Check sheet for the modelled part. Datum: model origin and axes. Units: mm. Face numbers are marked on the shaded views. A direction names the side the tool comes from. Give positions to 0.01 mm unless a question says otherwise; leave off trailing zeros. Write each loop counter-clockwise with the first axis right and the second up, starting at its lowest first coordinate (ties: lowest second). Pieces come first, ordered by that corner, then holes. Notation, with made-up numbers: M 61.5,-19 L 99.5,-19 A10 cw 99.5,0 Z; hole C -34,-13 d8. An arc over 180 degrees is marked long. Use CSV: the item, a comma, the result in double quotes. Start each with the question number.
1. Cross-section at C-C, the plane y = 12. Enter the section's corners in (x, z).
2. Cross-section at B-B, the plane x = 9. Enter the section's corners in (y, z).
3. Depth check by flat-ended pin: P1, Ø7.5, axis at x = -22.5, y = 13.5, coming from the +Z side; P2, Ø0.9, axis at x = -9, z = -18, coming from the +Y side; P3, Ø2.5, axis at x = -9.85, z = -18.519, coming from the -Y side; P4, Ø2, axis at y = -6.547, z = -15, coming from the -X side. Enter the tip coordinate at first touch or a pass-through.
4. Mould release check, pull along Z, two halves, no side actions. Record for the marked faces 6, 7, 8 and 9: +Z half, -Z half, draft (parallel to the pull), parting line (faces both ways), or undercut.
5. Access from +Z, -Z, +X, -X, +Y, -Y to the whole of each face (thin tool, end or side, straight path). Record for the marked faces 1, 2, 3, 4 and 5.
6. Cross-section at D-D, the plane y = -3.5. Enter the section's corners in (x, z).
7. Scan lines: line 1 (X direction, y = 2.45, z = -15); line 2 (X direction, y = 35.5, z = -11); line 3 (Y direction, x = -23, z = -21). Record each from-to range of solid material in increasing order.
8. Cross-section at A-A, the plane x = -17. Enter the section's corners in (y, z).
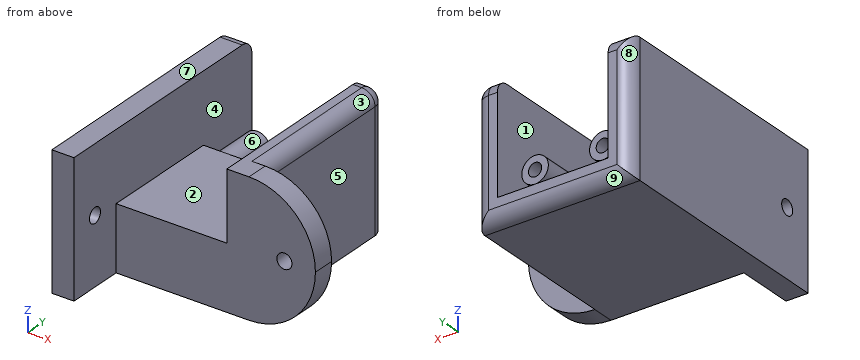
Autodesk Inventor part; units mm, degrees
ref_plane "YZ Plane" through (0, 0, 0) normal (1, 0, 0) x (0, 1, 0)
ref_plane "XZ Plane" through (0, 0, 0) normal (0, 1, 0) x (-1, 0, 0)
ref_plane "XY Plane" through (0, 0, 0) normal (0, 0, 1) x (1, 0, 0)
sketch "Sketch1" plane through (0, 0, 0) normal (0, 1, 0) x (-1, 0, 0)
  line L0 (0, 0) -> (35, 0) construction
  line L1 (35, 0) -> (35, -30)
  line L2 (35, -30) -> (0, -30)
  line L3 (0, -30) -> (0, 0)
  line L4 (30, -25) -> (30, -5)
  line L5 (30, -5) -> (5, -5) construction
  line L6 (5, -5) -> (5, -25)
  line L7 (5, -25) -> (30, -25)
  line L8 (30, -5) -> (30, 0)
  line L9 (5, -5) -> (5, 0)
  line L10 (5, 0) -> (0, 0)
  line L11 (30, 0) -> (35, 0)
  dimension "d0" = 35
  dimension "d1" = 30
  dimension "d2" = 5
extrude "Extrusion1" add sketch "Sketch1" along normal blind 42
sketch "Sketch2" plane through (0, 0, 0) normal (0, 1, 0) x (-1, 0, 0)
  line L0 (30, 0) -> (30, -25)
  line L1 (5, -25) -> (5, 0)
  line L2 (30, -25) -> (5, -25)
  line L3 (5, -25) -> (5, -15.519)
  line L4 (5, -15.519) -> (30, -15.519)
  line L5 (30, -15.519) -> (30, -25)
  point P0 (0, 0)
  dimension "d5" = 9.481
extrude "Extrusion2" add sketch "Sketch2" along normal blind 27
sketch "Sketch3" plane through (0, 27, 0) normal (0, 1, 0) x (1, 0, 0)
  circle A0 centre (-25.15, 18.519) radius 1.5
  line L0 (-30, 0) -> (-30, 15.519)
  circle A1 centre (-25.15, 18.519) radius 3
  line L1 (-30, 15.519) -> (-5, 15.519)
  line L2 (-17.5, 15.519) -> (-17.5, 30) construction
  line L3 (0, 30) -> (-35, 30) construction
  circle A2 centre (-9.85, 18.519) radius 1.5
  circle A3 centre (-9.85, 18.519) radius 3
  point P0 (0, 0)
  dimension "d8" = 3
  dimension "d9" = 4.85
  dimension "d10" = 6
extrude "Extrusion3" add sketch "Sketch3" along normal blind 10
sketch "Sketch4" plane through (0, 0, 0) normal (0, -1, 0) x (1, 0, 0)
  line L0 (-35, -30) -> (-35, 0)
  line L1 (0, -30) -> (-35, -30)
  line L2 (-35, 0) -> (-30, 0)
  line L3 (-30, 0) -> (-30, -30)
  line L4 (-30, -30) -> (-35, -30)
  line L5 (-35, -30) -> (-35, 0)
  line L6 (-30, 0) -> (-30, -15.519)
  point P0 (0, 0)
extrude "Extrusion4" add sketch "Sketch4" along normal blind 13.047
sketch "Sketch5" plane through (0, 0, 0) normal (1, 0, 0) x (0, 0, -1)
  line L0 (15.519, 0) -> (0, 0)
  line L1 (30, 0) -> (30, 42)
  line L2 (0, 0) -> (30, 0)
  line L3 (30, 0) -> (30, 5)
  line L4 (30, 5) -> (0, 5)
  line L5 (0, 5) -> (0, 0)
  dimension "d15" = 5
extrude "Extrusion5" add sketch "Sketch5" along normal blind 15
sketch "Sketch6" plane through (0, 5, 0) normal (0, 1, 0) x (1, 0, 0)
  circle A0 centre (8, 7) radius 3.5 construction
  circle A1 centre (8, 23) radius 3.5 construction
  line L0 (8, 7) -> (8, 23) construction
  line L1 (8, 15) -> (15, 15) construction
  line L2 (15, 0) -> (15, 30) construction
  line L3 (15, 30) -> (15, 0) construction
  line L4 (0, 30) -> (15, 30) construction
  circle A2 centre (8, 15) radius 1.7
  point P0 (0, 0)
  dimension "d18" = 7
  dimension "d19" = 7
  dimension "d20" = 7
  dimension "d21" = 7
  dimension "d25" = 3.4
extrude "Extrusion6" cut sketch "Sketch6" against normal up to surface (5 mm away) from surface at 0
sketch "Sketch7" plane through (-35, 42, -30) normal (-1, 0, 0) x (0, 0, 1)
  point P0 (30, -42)
sketch "Sketch8" plane through (-35, 42, -30) normal (-1, 0, 0) x (0, 0, 1)
  line L0 (0, -55.047) -> (0, 0)
  line L1 (30, -55.047) -> (30, 0)
  line L2 (0, -55.047) -> (30, -55.047) construction
  line L3 (30, -55.047) -> (30, -42.047) construction
  line L4 (30, -42.047) -> (0, -42.047) construction
  line L5 (0, -42.047) -> (0, -55.047) construction
  circle A0 centre (15, -48.547) radius 1.7
  point P0 (30, -42)
  dimension "d24" = 13
  dimension "d26" = 3.4
  dimension "d27" = 6.5
  dimension "d28" = 15
extrude "Extrusion7" cut sketch "Sketch8" against normal up to next
fillet "Fillet1" radius 3 6 edges at (0, 42, -15) (0, 23.5, 0) (-35, 42, -15) (-17.5, 42, -30) (-2.5, 42, 0) (-32.5, 42, 0)
fillet "Fillet2" radius 15 2 edges at (15, 2.5, 0) (15, 2.5, -30)
equation "\"d21\" = d20"
properties part number "imu_mount"
Worked answers:
1,outline,"M -35,-30 L 0,-30 L 0,-3 A3 ccw -3,0 L -5,0 L -5,-15.52 L -30,-15.52 L -30,0 L -35,0 Z"
2,outline,"M 0,-27 L 5,-27 L 5,-16.37 L 0,-16.37 Z; M 0,-13.63 L 5,-13.63 L 5,-3 L 0,-3 Z"
3,P1,"stops at z = -15.52"
3,P2,"stops at y = 27"
3,P3,"stops at y = 0"
3,P4,"passes through"
4,face 6,"undercut"
4,face 7,"+Z half"
4,face 8,"draft"
4,face 9,"-Z half"
5,face 1,"+Z, +Y"
5,face 2,"+Z, +Y, -Y"
5,face 3,"+Z, +X, +Y"
5,face 4,"+Z"
5,face 5,"+Z, -Z, +X, +Y"
6,outline,"M -35,-30 L -30,-30 L -30,0 L -35,0 Z"
7,line 1,"x = -35 to -30, -5 to 6.3, 9.7 to 15"
7,line 2,"x = -35 to -30, -5 to 0"
7,line 3,"y = 0 to 27"
8,outline,"M 0,-30 L 39,-30 A3 ccw 42,-27 L 42,-25 L 27,-25 L 27,-15.52 L 0,-15.52 Z"
